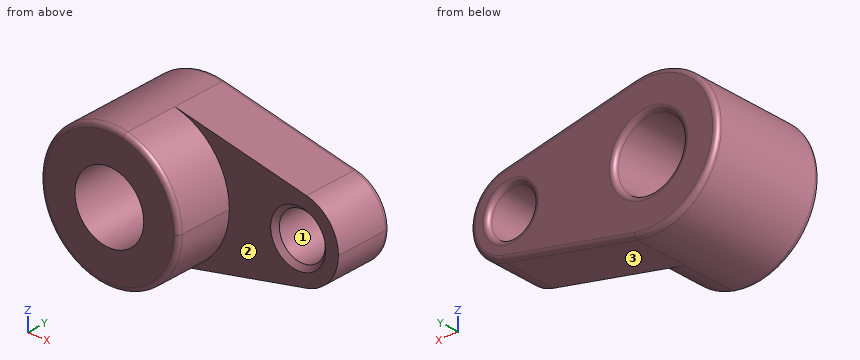
```python
from build123d import *

# Parameters (mm, degrees)
F0_R     = 38.1
F0_R_2   = 25.4
F1_DEPTH = 63.5
F2_DEPTH = 127
F3_R     = 5.08
F4_SIZE  = 5.08


with BuildPart() as f1:
    # F0 (on Front) → F1 (new body)
    with BuildSketch(Plane.XZ):
        with BuildLine():
            ThreePointArc((15.875, -74.528011), (59.228857, -47.941449), (76.2, 0))
            ThreePointArc((76.2, 0), (59.228857, 47.941449), (15.875, 74.528011))
            ThreePointArc((15.875, 74.528011), (-76.2, 0), (15.875, -74.528011))
        make_face()
        Circle(F0_R, mode=Mode.SUBTRACT)
        with BuildLine():
            ThreePointArc((15.875, 74.528011), (59.228857, 47.941449), (76.2, 0))
            ThreePointArc((76.2, 0), (59.228857, -47.941449), (15.875, -74.528011))
            Line((15.875, -74.528011), (161.660417, -43.474673))
            ThreePointArc((161.660417, -43.474673), (107.95, 0), (161.660417, 43.474673))
            Line((161.660417, 43.474673), (15.875, 74.528011))
        make_face()
        with BuildLine():
            ThreePointArc((196.85, 0), (186.950167, 27.965845), (161.660417, 43.474673))
            ThreePointArc((161.660417, 43.474673), (107.95, 0), (161.660417, -43.474673))
            ThreePointArc((161.660417, -43.474673), (186.950167, -27.965845), (196.85, 0))
        make_face()
        with Locations((152.4, 0)):
            Circle(F0_R_2, mode=Mode.SUBTRACT)
    extrude(amount=F1_DEPTH)

    # F0 (on Front) → F2 (join)
    with BuildSketch(Plane.XZ):
        with BuildLine():
            ThreePointArc((15.875, -74.528011), (59.228857, -47.941449), (76.2, 0))
            ThreePointArc((76.2, 0), (59.228857, 47.941449), (15.875, 74.528011))
            ThreePointArc((15.875, 74.528011), (-76.2, 0), (15.875, -74.528011))
        make_face()
        Circle(F0_R, mode=Mode.SUBTRACT)
    extrude(amount=F2_DEPTH)

    # F3
    f3_edges = [f1.edges().sort_by_distance(p)[0] for p in [
        (-15.875, -127, 74.528011),
        (-76.2, 0, 0),
        (88.767708, 0, -59.001342),
        (196.85, 0, 0),
        (88.767708, 0, 59.001342),
        (-38.1, 0, 0),
        (127, 0, 0),
    ]]
    fillet(f3_edges, radius=F3_R)

    # F4
    f4_edges = [f1.edges().sort_by_distance(p)[0] for p in [
        (127, -63.5, 0),
    ]]
    chamfer(f4_edges, length=F4_SIZE)


solid = f1.part
```
Could you check a few things on this model? Use its own coordinates, in mm. Face numbers are marked on the shaded views. Round coordinates to 2 decimals unless told otherwise and drop trailing zeros. Write each loop counter-clockwise with the first axis right and the second up, starting at its lowest first coordinate (ties: lowest second). Pieces come first, ordered by that corner, then holes. Notation, with made-up numbers: M 7.5,52.25 L 66.5,52.25 A10 ccw 66.5,59.25 Z; hole C -17,-39 d6. An arc over 180 degrees is marked long. Answer in a Markdown table with one row per item. Add a question column.
Q1. Imagine slicing it at C-C (y = -105.5). Please give me the cut outline in (x, z) (3 decimals), then the cut area to 3 significant figures.
Q2. If we mould it in two halves opening along Z, with no side actions, what happens to the marked faces 1, 2 and 3? For each: +Z half, -Z half, draft (parallel to the pull), parting line (faces both ways), or undercut.
Q3. Imagine slicing it at B-B (z = -5.5). Give the number of separate pieces and of enclosed holes in the cut face, then the cut area to 3 significant figures.
Q4. Will these pins go through, and if not, where does the flat tip stop? pin 1 Ø4 at (x, y) = (121.5, -30.5) entering from +Z; pin 2 Ø12 at (y, z) = (-75.5, 27.5) entering from -X; pin 3 Ø10 at (x, z) = (127.5, -3.5) entering from -Y.
Q5. Imagine slicing it at A-A (y = -26.5). Please give me the cut outline in (x, z) (3 decimals), then the cut area to 3 significant figures.
Q6. If I drill on line 1 (Z direction, x = 0, y = -100); line 2 (X direction, y = -55.5, z = -6.5); line 3 (Z direction, x = 152, y = -32), over which ranges is the centre line in solid material (lowest first)? Write a range as from..to.
Values:
| question | item | result |
|---|---|---|
| 1 | outline | C 0,0 d152.4; hole C 0,0 d76.2 |
| 1 | area | 13,700 mm^2 |
| 2 | face 1 | undercut |
| 2 | face 2 | draft |
| 2 | face 3 | -Z half |
| 3 | separate pieces | 3 |
| 3 | enclosed holes | 0 |
| 3 | area | 14,200 mm^2 |
| 4 | pin 1 | z = 52.46 |
| 4 | pin 2 | x = -73.1 |
| 4 | pin 3 | y = -63.16 |
| 5 | outline | M 15.875,-74.528 L 161.66,-43.475 A44.45 ccw 196.85,0 A44.45 ccw 161.66,43.475 L 15.875,74.528 A76.2 ccw long Z; hole C 0,0 d76.2; hole C 152.4,0 d50.8 |
| 5 | area | 24,400 mm^2 |
| 6 | line 1 | -76.2..-38.1, 38.1..76.2 |
| 6 | line 2 | -75.92..-37.54, 37.54..127.85, 176.95..196.37 |
| 6 | line 3 | -45.53..-25.4, 25.4..45.53 |
